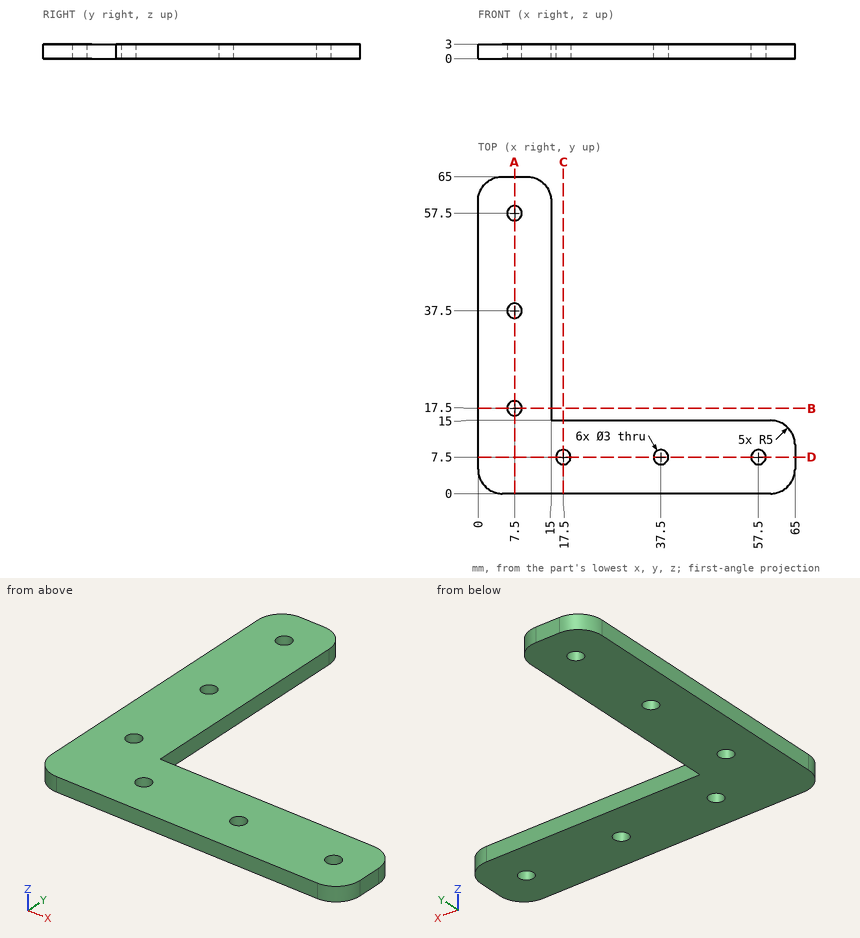
Study the drawing (mm; zero at the part's minimum x, y, z) and answer. Round coordinates to 2 decimals unless told otherwise and drop trailing zeros. Write each loop counter-clockwise with the first axis right and the second up, starting at its lowest first coordinate (ties: lowest second). Pieces come first, ordered by that corner, then holes. Notation, with made-up numbers: (65.5, 88) -> (122.5, 88) arc R16 ccw to (122.5, 101) -> close; hole circle Ø4 at (41, 33.25). An arc over 180 degrees is marked (long way). Use CSV: the item, a comma, the result in double quotes. Start each with the question number.
(1) Section B-B on y = 17.5 is taken. Give the vertices of the cut face in (x, z), then the cut area to 3 significant figures.
(2) Consider L1, parallel to Y at x = 7.5, z = 2.4; L2, parallel to Y at x = 36.5, z = 1.95; L3, parallel to X at y = 35, z = 0.25. Determine where each line is inside the solid, lowest interval first. Write a range as from..to.
(3) Each of these flat-tipped pins is pushed along its axis until it touches: pin 1 (0.9 mm diameter, centred on x = 36, z = 1.5, fed in from +Y); pin 2 (1.5 mm diameter, centred on y = 46.5, z = 2, fed in from +X). Where does it stop, or does it pass through?
(4) Section A-A on x = 7.5 is taken. Give the vertices of the cut face in (y, z), then the cut area to 3 significant figures.
A:
1,outline,"(0, 0) -> (6, 0) -> (6, 3) -> (0, 3) -> close; (9, 0) -> (15, 0) -> (15, 3) -> (9, 3) -> close"
1,area,"36.0 mm²"
2,L1,"y = 0..16, 19..36, 39..56, 59..65"
2,L2,"y = 0..6.38, 8.62..15"
2,L3,"x = 0..15"
3,pin 1,"stops at y = 15"
3,pin 2,"stops at x = 15"
4,outline,"(0, 0) -> (16, 0) -> (16, 3) -> (0, 3) -> close; (19, 0) -> (36, 0) -> (36, 3) -> (19, 3) -> close; (39, 0) -> (56, 0) -> (56, 3) -> (39, 3) -> close; (59, 0) -> (65, 0) -> (65, 3) -> (59, 3) -> close"
4,area,"168 mm²"
